CAD build for the part. Positions are in the model's coordinates, mm. Round coordinates to 2 decimals unless told otherwise and drop trailing zeros. Order: outer loops, then holes, each group sorted by start corner. A loop starts at its lowest first (then second) coordinate and runs counter-clockwise, first axis right, second up.
```python
from build123d import *

# Parameters (mm, degrees)
F0_W      = 1840
F0_H      = 750
F1_DEPTH  = 25
F2_W      = 1790
F2_H      = 25
F3_DEPTH  = 25
F5_DEPTH  = 65
F7_W      = 25
F7_H      = 25
F8_DEPTH  = 675
F10_DEPTH = 65
F12_W     = 25
F12_H     = 25
F13_DEPTH = 675
F15_W     = 25
F15_H     = 25
F16_DEPTH = 675
F18_W     = 25
F18_H     = 25
F19_DEPTH = 650
F21_W     = 25
F21_H     = 25
F22_DEPTH = 650
F24_DEPTH = 10
F26_DEPTH = 10
F28_DEPTH = 10
F30_DEPTH = 10


with BuildPart() as f1:
    # F0 (on Top) → F1 (new body)
    with BuildSketch(Plane.XY):
        with Locations((-920, 375)):
            Rectangle(F0_W, F0_H)
    extrude(amount=F1_DEPTH)

    # F2 (on face) → F3 (join)
    with BuildSketch(Plane(origin=(0, 0, 0), x_dir=(1, 0, 0), z_dir=(0, 0, -1))):
        with Locations((-920, -37.5)):
            Rectangle(F2_W, F2_H)
        with Locations((-920, -712.5)):
            Rectangle(F2_W, F2_H)
    extrude(amount=F3_DEPTH)

    # F4 (on face) → F5 (join)
    with BuildSketch(Plane(origin=(0, 0, 0), x_dir=(1, 0, 0), z_dir=(0, 0, -1))):
        Polygon((-65, -25), (-25, -25), (-25, -50), (-65, -50), (-65, -52), (-23, -52), (-23, -23), (-65, -23), align=None)
    extrude(amount=F5_DEPTH)

    # F7 (on offset) → F8 (join)
    with BuildSketch(Plane(origin=(0, 0, -35), x_dir=(1, 0, 0), z_dir=(0, 0, -1))):
        with Locations((-37.5, -37.523640207)):
            Rectangle(F7_W, F7_H)
    extrude(amount=F8_DEPTH)

    # F9 (on face) → F10 (join)
    with BuildSketch(Plane.XY):
        Polygon((-1815, 725), (-1775, 725), (-1775, 727), (-1817, 727), (-1817, 698), (-1775, 698), (-1775, 700), (-1815, 700), align=None)
        Polygon((-65.0490959734, 726.9829173088), (-65.0490959734, 724.9829173088), (-25.0490959734, 724.9829173088), (-25.0490959734, 699.9829173088), (-65.0490959734, 699.9829173088), (-65.0490959734, 697.9829173088), (-23.0490959734, 697.9829173088), (-23.0490959734, 726.9829173088), align=None)
        Polygon((-1775, 25), (-1815, 25), (-1815, 50), (-1775, 50), (-1775, 52), (-1817, 52), (-1817, 23), (-1775, 23), align=None)
    extrude(amount=-F10_DEPTH)

    # F12 (on offset) → F13 (join)
    with BuildSketch(Plane(origin=(0, 0, -35), x_dir=(1, 0, 0), z_dir=(0, 0, -1))):
        with Locations((-1802.5, -37.5)):
            Rectangle(F12_W, F12_H)
    extrude(amount=F13_DEPTH)

    # F15 (on offset) → F16 (join)
    with BuildSketch(Plane(origin=(0, 0, -35), x_dir=(1, 0, 0), z_dir=(0, 0, -1))):
        with Locations((-37.5, -712.5)):
            Rectangle(F15_W, F15_H)
        with Locations((-1802.5, -712.5)):
            Rectangle(F15_W, F15_H)
    extrude(amount=F16_DEPTH)

    # F18 (on offset) → F19 (join)
    with BuildSketch(Plane(origin=(0, 50.023640207, 0), x_dir=(-1, 0, 0), z_dir=(0, 1, 0))):
        with Locations((37.5, -497.5)):
            Rectangle(F18_W, F18_H)
    extrude(amount=F19_DEPTH)

    # F21 (on offset) → F22 (join)
    with BuildSketch(Plane(origin=(0, 50, 0), x_dir=(-1, 0, 0), z_dir=(0, 1, 0))):
        with Locations((1802.5, -497.5)):
            Rectangle(F21_W, F21_H)
    extrude(amount=F22_DEPTH)

    # F23 (on face) → F24 (join)
    with BuildSketch(Plane.XZ.offset(-700)):
        with BuildLine():
            Line((-50, -188.7835379987), (-236.028425198, -5.3788918093))
            ThreePointArc((-236.028425198, -5.3788918093), (-249.6380961216, -4.9776946987), (-251.0328083047, -18.5216557034))
            Line((-251.0328083047, -18.5216557034), (-50, -216.7190604298))
            Line((-50, -216.7190604298), (-50, -188.7835379987))
        make_face()
        with BuildLine():
            Line((-29.5162876687, -208.9783442966), (-50, -188.7835379987))
            Line((-50, -188.7835379987), (-50, -216.7190604298))
            Line((-50, -216.7190604298), (-44.5206707754, -222.1211081907))
            ThreePointArc((-44.5206707754, -222.1211081907), (-30.9109998517, -222.5223053013), (-29.5162876687, -208.9783442966))
        make_face()
    extrude(amount=F24_DEPTH)

    # F25 (on face) → F26 (join)
    with BuildSketch(Plane(origin=(0, 50.023640207, 0), x_dir=(-1, 0, 0), z_dir=(0, 1, 0))):
        with BuildLine():
            Line((50, -188.6229664357), (50, -216.7160920101))
            Line((50, -216.7160920101), (250.9788283543, -18.4630064225))
            ThreePointArc((250.9788283543, -18.4630064225), (251.07538107, -4.3212004002), (236.9335750477, -4.2246476845))
            Line((236.9335750477, -4.2246476845), (50, -188.6229664357))
        make_face()
        with BuildLine():
            ThreePointArc((30.4773733467, -207.880820631), (30.380820631, -222.0226266533), (44.5226266533, -222.119179369))
            Line((44.5226266533, -222.119179369), (50, -216.7160920101))
            Line((50, -216.7160920101), (50, -188.6229664357))
            Line((50, -188.6229664357), (30.4773733467, -207.880820631))
        make_face()
    extrude(amount=F26_DEPTH)

    # F27 (on face) → F28 (join)
    with BuildSketch(Plane(origin=(0, 50, 0), x_dir=(-1, 0, 0), z_dir=(0, 1, 0))):
        with BuildLine():
            ThreePointArc((1792.287088182, -222.1476128693), (1806.4283860793, -221.993685028), (1806.274458238, -207.8523871307))
            Line((1806.274458238, -207.8523871307), (1790, -191.9284084544))
            Line((1790, -191.9284084544), (1790, -219.9097784106))
            Line((1790, -219.9097784106), (1792.287088182, -222.1476128693))
        make_face()
        with BuildLine():
            Line((1790, -219.9097784106), (1790, -191.9284084544))
            Line((1790, -191.9284084544), (1598.993685028, -5.0355213195))
            ThreePointArc((1598.993685028, -5.0355213195), (1584.8523871307, -5.1894491609), (1585.006314972, -19.3307470582))
            Line((1585.006314972, -19.3307470582), (1790, -219.9097784106))
        make_face()
    extrude(amount=F28_DEPTH)

    # F29 (on face) → F30 (join)
    with BuildSketch(Plane.XZ.offset(-700)):
        with BuildLine():
            Line((-1599.022452861, -5.0670719967), (-1790, -191.924401237))
            Line((-1790, -191.924401237), (-1790, -219.9052243348))
            Line((-1790, -219.9052243348), (-1585.0408926577, -19.3679780711))
            ThreePointArc((-1585.0408926577, -19.3679780711), (-1584.8839824349, -5.2294459524), (-1599.022452861, -5.0670719967))
        make_face()
        with BuildLine():
            Line((-1790, -191.924401237), (-1806.3072462202, -207.8798290955))
            ThreePointArc((-1806.3072462202, -207.8798290955), (-1806.4641564431, -222.0183612143), (-1792.325686017, -222.1807351699))
            Line((-1792.325686017, -222.1807351699), (-1790, -219.9052243348))
            Line((-1790, -219.9052243348), (-1790, -191.924401237))
        make_face()
    extrude(amount=F30_DEPTH)


solid = f1.part
```
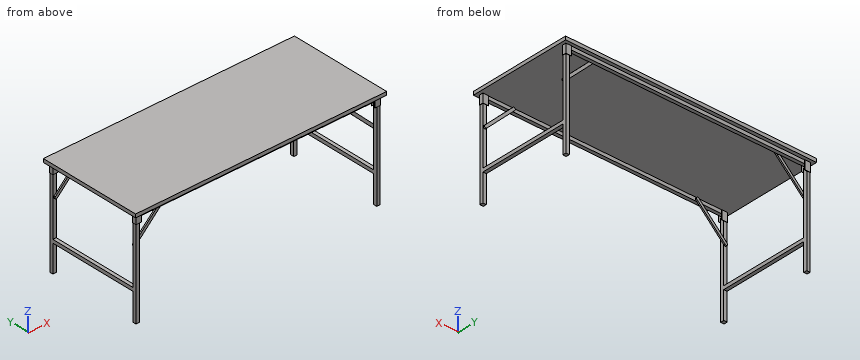
1. Cut at A-A, the plane y = 636.5. Write the cut outline in (x, z).
2. Pin check, flat tips, straight feed: P1, Ø7.5, axis at y = 717.5, z = -22, coming from the -X side; P2, Ø7.5, axis at x = -31.5, z = -276, coming from the +Y side; P3, Ø0.6, axis at y = 24, z = -26.5, coming from the +X side. Stop position of each tip, or through.
3. Cut at C-C, the plane x = -1512.5. Write the cut outline in (y, z).
4. Cut at B-B, the plane z = -625. Write the cut outline in (x, y).
5. Cut at D-D, the plane x = -159. Write the cut outline in (y, z), and give its area (3 significant figures).
6. Drill centre lines: line 1 (Z direction, x = -732.5, y = 686); line 2 (X direction, y = 716, z = -131); line 3 (Z direction, x = -1598, y = 691.5). Where is each one in solid material? Low to high.
Outcome:
1. outline: (-1840, 0) - (0, 0) - (0, 25) - (-1840, 25) - close; (-1815, -510) - (-1790, -510) - (-1790, -485) - (-1815, -485) - close; (-50, -510) - (-25, -510) - (-25, -485) - (-50, -485) - close
2. P1: stops at x = -1817
2. P2: stops at y = 725
2. P3: stops at x = -23
3. outline: (0, 0) - (25, 0) - (25, -25) - (50, -25) - (50, 0) - (700, 0) - (700, -25) - (725, -25) - (725, 0) - (750, 0) - (750, 25) - (0, 25) - close
4. outline: (-1815, 25) - (-1790, 25) - (-1790, 50) - (-1815, 50) - close; (-1815, 700) - (-1790, 700) - (-1790, 725) - (-1815, 725) - close; (-50, 25.02) - (-25, 25.02) - (-25, 50.02) - (-50, 50.02) - close; (-50, 700) - (-25, 700) - (-25, 725) - (-50, 725) - close
5. outline: (0, 0) - (25, 0) - (25, -25) - (50, -25) - (50, 0) - (700, 0) - (700, -25) - (725, -25) - (725, 0) - (750, 0) - (750, 25) - (0, 25) - close; (50.02, -109.19) - (60.02, -109.19) - (60.02, -81.1) - (50.02, -81.1) - close; (690, -109.26) - (700, -109.26) - (700, -81.32) - (690, -81.32) - close
5. area: 20,600 mm2
6. line 1: z = 0 to 25
6. line 2: x = -1815 to -1790, -50 to -25
6. line 3: z = -32.05 to -4.19, 0 to 25
